```python
from build123d import *

# Parameters (mm, degrees)
F0_R     = 4.5
F0_R_2   = 1.185
F1_DEPTH = 3
F0_R_3   = 2
F2_DEPTH = 4.5


with BuildPart() as f1:
    # F0 (on Top) → F1 (new body)
    with BuildSketch(Plane.XY):
        with BuildLine():
            Line((-3, 12.134661), (-9.06962, -8.60186))
            ThreePointArc((-9.06962, -8.60186), (0, -12.5), (9.06962, -8.60186))
            Line((9.06962, -8.60186), (3, 12.134661))
            ThreePointArc((3, 12.134661), (0, 12.5), (-3, 12.134661))
        make_face()
        Circle(F0_R, mode=Mode.SUBTRACT)
        with Locations((0, 9)):
            Circle(F0_R_2, mode=Mode.SUBTRACT)
    extrude(amount=F1_DEPTH)

    # F0 (on Top) → F2 (join)
    with BuildSketch(Plane.XY):
        Circle(F0_R)
        Circle(F0_R_3, mode=Mode.SUBTRACT)
    extrude(amount=F2_DEPTH)


solid = f1.part
```
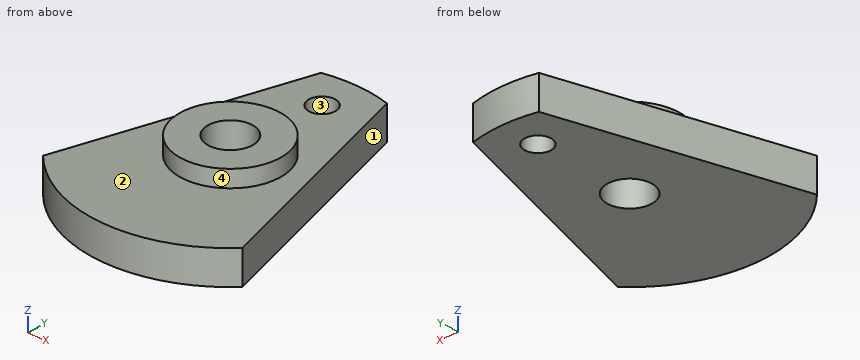
Geometry check sheet. Reference: the model listing, model coordinates, mm. Face numbers are marked on the shaded views. Give positions to 0.01 mm unless a question says otherwise; leave off trailing zeros. Loops run counter-clockwise (first coordinate to the right, second up) from the corner with the lowest first, then second, coordinate; pieces in that order, holes last. Notation, with made-up numbers: (29, 62) - (72, 62) arc R34 ccw to (72, 95) - close; hole circle Ø11 at (80, 74.5). An arc over 180 degrees is marked (long way). Use CSV: the item, a comma, the result in double quotes. Start each with the question number.
Q1. Go/stop test with flat-tipped pins: pin 1 Ø2 at (x, z) = (3.5, 3) entering from -Y; pin 2 Ø5 at (x, y) = (0, -8.5) entering from +Z; pin 3 Ø2.5 at (x, y) = (0, 0) entering from -Z. Record where each tip stops, or that it passes through.
Q2. Section check B-B, the plane y = -1. Record the cut outline in (x, z).
Q3. Release check for a two-part mould opening along Y. For the marked faces 1, 2, 3 and 4 record: +Y half, -Y half, draft (parallel to the pull), parting line (faces both ways), or undercut.
Q4. Section check A-A, the plane x = 0. Record the cut outline in (y, z) (3 decimals).
Q5. Section check D-D, the plane y = 3.5. Record the cut outline in (x, z), and give its area (3 significant figures).
Q6. Section check C-C, the plane z = 2. Record the cut outline in (x, y) (3 decimals), and give its area (3 significant figures).
Q7. Scan lines: probe 1 along Y at (x, z) = (0, 1.2) (3 decimals); probe 2 along Y at (x, z) = (0, 3.1); probe 3 along Z at (x, y) = (-1.5, 10.25). Record each from-to range of solid material in increasing order. Write a range as from..to.
Findings below:
1,pin 1,"stops at y = -12.25"
1,pin 2,"stops at z = 3"
1,pin 3,"passes through"
2,outline,"(-6.84, 0) - (-1.73, 0) - (-1.73, 4.5) - (-4.39, 4.5) - (-4.39, 3) - (-6.84, 3) - close; (1.73, 0) - (6.84, 0) - (6.84, 3) - (4.39, 3) - (4.39, 4.5) - (1.73, 4.5) - close"
3,face 1,"+Y half"
3,face 2,"draft"
3,face 3,"undercut"
3,face 4,"parting line"
4,outline,"(-12.5, 0) - (-2, 0) - (-2, 4.5) - (-4.5, 4.5) - (-4.5, 3) - (-12.5, 3) - close; (2, 0) - (7.815, 0) - (7.815, 3) - (4.5, 3) - (4.5, 4.5) - (2, 4.5) - close; (10.185, 0) - (12.5, 0) - (12.5, 3) - (10.185, 3) - close"
5,outline,"(-5.53, 0) - (5.53, 0) - (5.53, 3) - (2.83, 3) - (2.83, 4.5) - (-2.83, 4.5) - (-2.83, 3) - (-5.53, 3) - close"
5,area,"41.6 mm^2"
6,outline,"(-9.07, -8.602) arc R12.5 ccw to (9.07, -8.602) - (3, 12.135) arc R12.5 ccw to (-3, 12.135) - close; hole circle Ø4 at (0, 0); hole circle Ø2.37 at (0, 9)"
6,area,"284 mm^2"
7,probe 1,"y = -12.5..-2, 2..7.815, 10.185..12.5"
7,probe 2,"y = -4.5..-2, 2..4.5"
7,probe 3,"z = 0..3"
